Read the model definition and answer for the solid it produces. Units are mm, in the model's axes. A direction names the side the tool comes from. Coordinates: 2 decimals unless noted, no trailing zeros. Order: outer loops, then holes, each group sorted by start corner. A loop starts at its lowest first (then second) coordinate and runs counter-clockwise, first axis right, second up. Notation, with made-up numbers: (53.25, 80) - (66.25, 80) arc R29 ccw to (66.25, 117) - close; hole circle Ø8 at (15, 23.25). An arc over 180 degrees is marked (long way). Use one line per item in the form item = value. Start each with the question number.
from build123d import *

# Parameters (mm, degrees)
SKETCH1_W               = 50
SKETCH1_H               = 3
SKETCH2_W               = 12
SKETCH2_H               = 0.75
CUT_EXTRUDE1_DEPTH      = 4
CUT_EXTRUDE1_DEPTH_BACK = 4
SKETCH3_R               = 1.1
CUT_EXTRUDE2_DEPTH      = 4
CUT_EXTRUDE2_DEPTH_BACK = 4


with BuildPart() as part:
    # Sketch1 → Revolve1 (revolve)
    with BuildSketch(Plane.XY):
        with Locations((0, 1.5)):
            Rectangle(SKETCH1_W, SKETCH1_H)
    revolve(axis=Axis((0, 0, 0), (1, 0, 0)))

    # Sketch2 → Cut-Extrude1 (cut, two sides)
    with BuildSketch(Plane.XY) as cut_extrude1_sk:
        with Locations((-19, 2.625)):
            Rectangle(SKETCH2_W, SKETCH2_H)
        with Locations((-19, -2.625)):
            Rectangle(SKETCH2_W, SKETCH2_H)
        with Locations((19, 2.625)):
            Rectangle(SKETCH2_W, SKETCH2_H)
        with Locations((19, -2.625)):
            Rectangle(SKETCH2_W, SKETCH2_H)
    extrude(amount=CUT_EXTRUDE1_DEPTH, mode=Mode.SUBTRACT)
    extrude(cut_extrude1_sk.sketch, amount=-CUT_EXTRUDE1_DEPTH_BACK, mode=Mode.SUBTRACT)

    # Sketch3 → Cut-Extrude2 (cut, two sides)
    with BuildSketch(Plane.XY) as cut_extrude2_sk:
        with Locations((-20, 0)):
            Circle(SKETCH3_R)
        with Locations((20, 0)):
            Circle(SKETCH3_R)
    extrude(amount=CUT_EXTRUDE2_DEPTH, mode=Mode.SUBTRACT)
    extrude(cut_extrude2_sk.sketch, amount=-CUT_EXTRUDE2_DEPTH_BACK, mode=Mode.SUBTRACT)


solid = part.part
Q1. Consider probe 1 along X at (y, z) = (0, -0.25); probe 2 along Y at (x, z) = (20, 1.9); probe 3 along X at (y, z) = (-0.75, 2). Determine where each line is inside the solid, lowest interval first.
Q2. A cutting plane is placed at C-C (z = -1.5). Give the vertices of the cut face in (x, y), then the cut area to 3 significant figures.
Q3. A cutting plane is placed at D-D (x = -9). Give the vertices of the cut face in (y, z).
Q4. Given P1, Ø1.2, axis at x = -20, z = 0.5, coming from the +Y side; P2, Ø0.6, axis at y = -2.5, z = 0, coming from the -X side; P3, Ø1.2, axis at x = -19, z = -1, coming from the -Y side, each flat-ended and moving along its own axis, determine where each tip first touches the part or whether it passes through.
Q5. A cutting plane is placed at B-B (x = -20). Give the vertices of the cut face in (y, z).
Q6. Which of the six approach directions +Z, -Z, +X, -X, +Y, -Y give full straight-line access (tool end or side, diameter ignored) to faces 1 (the flat face through (19, -2.25, 0)), 2 (the flat face through (19, 2.25, 0)), 3 (the flat face through (-19, 2.25, 0))?
Q7. A cutting plane is placed at A-A (y = 0). Give the vertices of the cut face in (x, z).
Result sheet:
q1.probe_1 = -25 to -21.1, -18.9 to 18.9, 21.1 to 25
q1.probe_2 = -2.25 to -1.1, 1.1 to 2.25
q1.probe_3 = -25 to -20.8, -19.2 to 19.2, 20.8 to 25
q2.outline = (-25, -2.25) - (-13, -2.25) - (-13, -2.6) - (13, -2.6) - (13, -2.25) - (25, -2.25) - (25, 2.25) - (13, 2.25) - (13, 2.6) - (-13, 2.6) - (-13, 2.25) - (-25, 2.25) - close; hole circle Ø2.2 at (-20, 0); hole circle Ø2.2 at (20, 0)
q2.area = 235 mm^2
q3.outline = circle Ø6 at (0, 0)
q4.P1 = 2.25
q4.P2 = -25
q4.P3 = -2.25
q5.outline = (-2.25, -1.98) arc R3 ccw to (-1.1, -2.79) - (-1.1, 2.79) arc R3 ccw to (-2.25, 1.98) - close; (1.1, -2.79) arc R3 ccw to (2.25, -1.98) - (2.25, 1.98) arc R3 ccw to (1.1, 2.79) - close
q6.face_1 = +Z, -Z, +X, -Y
q6.face_2 = +Z, -Z, +X, +Y
q6.face_3 = +Z, -Z, -X, +Y
q7.outline = (-25, -3) - (-21.1, -3) - (-21.1, 3) - (-25, 3) - close; (-18.9, -3) - (18.9, -3) - (18.9, 3) - (-18.9, 3) - close; (21.1, -3) - (25, -3) - (25, 3) - (21.1, 3) - close
